Model file for the job. Use its own axes, mm. Give positions to 0.01 mm unless a question says otherwise; leave off trailing zeros. Write each loop counter-clockwise with the first axis right and the second up, starting at its lowest first coordinate (ties: lowest second). Pieces come first, ordered by that corner, then holes. Notation, with made-up numbers: (77.5, 77) - (131.5, 77) arc R32 cw to (131.5, 104) - close; hole circle Ø9 at (-30.5, 5). An arc over 180 degrees is marked (long way). One line per item, written item: value. Start each with the question number.
(1) Cut at C-C, the plane x = -2.25. List the corners of the cut face in (y, z), and give its area (3 significant figures).
(2) Mould opens along Z. For faces 1 (the face through (0, 0, 6.792)), 2 (the face through (6.02, -6, 0)), 3 (the face through (0.084, -4.213, 3.864)), 4 (the face through (0, 0, -6.792)) say: pulls with the +Z half, pulls with the -Z half, needs draft (parallel to the pull), parting line crosses it, or undercut.
(3) Cut at A-A, the plane y = 0. List the corners of the cut face in (x, z).
(4) Probe L1, parallel to Z at x = 1, y = 0; L2, parallel to Y at x = -5, z = -2.25; L3, parallel to Y at x = 3.25, z = -3. List the from-to ranges inside material, lowest first.
(5) Cut at B-B, the plane z = 0. List the corners of the cut face in (x, y), and give its area (3 significant figures).
from build123d import *

# Parameters (mm, degrees)
F0_W          = 12.03933
F0_H          = 13.584534
F1_DEPTH      = 25.4
F1_DEPTH_BACK = 25.4
F2_R          = 5.716631
F3_DEPTH      = 25.4


with BuildPart() as f1:
    # F0 (on Front) → F1 (new body, two sides)
    with BuildSketch(Plane.XZ) as f1_sk:
        Rectangle(F0_W, F0_H)
    extrude(amount=F1_DEPTH)
    extrude(f1_sk.sketch, amount=-F1_DEPTH_BACK)

    # F2 (on face) → F3 (cut)
    with BuildSketch(Plane.YZ.offset(6.019665)):
        Circle(F2_R)
    extrude(amount=-F3_DEPTH, mode=Mode.SUBTRACT)


solid = f1.part
Answers follow:
1. outline: (-25.4, -6.79) - (25.4, -6.79) - (25.4, 6.79) - (-25.4, 6.79) - close; hole circle Ø11.43 at (0, 0)
1. area: 587 mm²
2. face 1: pulls with the +Z half
2. face 2: needs draft
2. face 3: undercut
2. face 4: pulls with the -Z half
3. outline: (-6.02, -6.79) - (6.02, -6.79) - (6.02, -5.72) - (-6.02, -5.72) - close; (-6.02, 5.72) - (6.02, 5.72) - (6.02, 6.79) - (-6.02, 6.79) - close
4. L1: z = -6.79 to -5.72, 5.72 to 6.79
4. L2: y = -25.4 to -5.26, 5.26 to 25.4
4. L3: y = -25.4 to -4.87, 4.87 to 25.4
5. outline: (-6.02, -25.4) - (6.02, -25.4) - (6.02, -5.72) - (-6.02, -5.72) - close; (-6.02, 5.72) - (6.02, 5.72) - (6.02, 25.4) - (-6.02, 25.4) - close
5. area: 474 mm²
